Geometry check sheet. Reference: drawing and pictorial views, mm from the part's lowest x, y, z. A direction names the side the tool comes from. Give positions to 0.01 mm unless a question says otherwise; leave off trailing zeros. Order: outer loops, then holes, each group sorted by start corner. A loop starts at its lowest first (then second) coordinate and runs counter-clockwise, first axis right, second up.
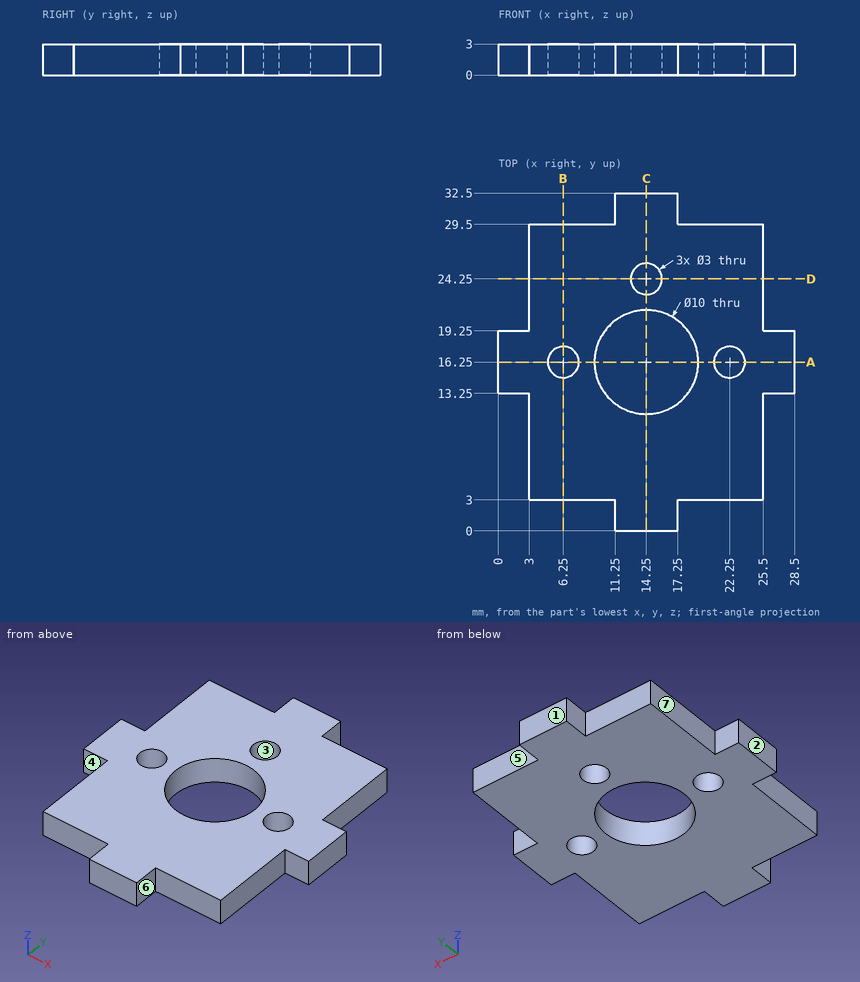
(1) Go/stop test with flat-tipped pins: P1, Ø0.9, axis at x = 27, z = 1, coming from the -Y side; P2, Ø1.5, axis at x = 7.5, z = 2, coming from the +Y side; P3, Ø1.5, axis at y = 9, z = 1.5, coming from the -X side. Record where each tip stops, or that it passes through.
(2) Sectioned sample at B-B (x = 6.25). Enter the section's corners in (y, z), plus the area to 3 significant figures.
(3) Thickness scan on L1, parallel to Y at x = 14.25, z = 2.45; L2, parallel to X at y = 17, z = 1.65; L3, parallel to Y at x = 22.25, z = 1.75. Record the ranges inside material, lowest first.
(4) Release check for a two-part mould opening along X. For the marked faces 1, 2 and 3 record: released by +X, released by -X, zero draft, split by the parting line, or undercut.
(5) Tool access check on the marked faces 4, 5, 6 and 7. Record the directions out of +Z, -Z, +X, -X, +Y, -Y that give a thin tool (end or side, any length) a straight path to the whole face; none if there is none.
(6) Sectioned sample at A-A (y = 16.25). Enter the section's corners in (x, z), plus the area to 3 significant figures.
(7) Sectioned sample at D-D (y = 24.25). Enter the section's corners in (x, z), plus the area to 3 significant figures.
(8) Sectioned sample at C-C (x = 14.25). Enter the section's corners in (y, z), plus the area to 3 significant figures.
Values follow:
1. P1: stops at y = 13.25
1. P2: stops at y = 29.5
1. P3: stops at x = 3
2. outline: (3, 0) - (14.75, 0) - (14.75, 3) - (3, 3) - close; (17.75, 0) - (29.5, 0) - (29.5, 3) - (17.75, 3) - close
2. area: 70.5 mm2
3. L1: y = 0 to 11.25, 21.25 to 22.75, 25.75 to 32.5
3. L2: x = 0 to 4.95, 7.55 to 9.31, 19.19 to 20.95, 23.55 to 28.5
3. L3: y = 3 to 14.75, 17.75 to 29.5
4. face 1: zero draft
4. face 2: released by -X
4. face 3: undercut
5. face 4: +Z, -Z, -X, -Y
5. face 5: +Z, -Z, +X, +Y
5. face 6: +Z, -Z, +X, -Y
5. face 7: +Z, -Z, -X, +Y
6. outline: (0, 0) - (4.75, 0) - (4.75, 3) - (0, 3) - close; (7.75, 0) - (9.25, 0) - (9.25, 3) - (7.75, 3) - close; (19.25, 0) - (20.75, 0) - (20.75, 3) - (19.25, 3) - close; (23.75, 0) - (28.5, 0) - (28.5, 3) - (23.75, 3) - close
6. area: 37.5 mm2
7. outline: (3, 0) - (12.75, 0) - (12.75, 3) - (3, 3) - close; (15.75, 0) - (25.5, 0) - (25.5, 3) - (15.75, 3) - close
7. area: 58.5 mm2
8. outline: (0, 0) - (11.25, 0) - (11.25, 3) - (0, 3) - close; (21.25, 0) - (22.75, 0) - (22.75, 3) - (21.25, 3) - close; (25.75, 0) - (32.5, 0) - (32.5, 3) - (25.75, 3) - close
8. area: 58.5 mm2
